```python
from build123d import *

# Parameters (mm, degrees)
SKETCH1_R           = 20
BOSS_EXTRUDE1_DEPTH = 35
CUT_EXTRUDE1_DEPTH  = 15
SKETCH3_R           = 4.1
CUT_EXTRUDE2_DEPTH  = 21
SKETCH4_R           = 2
CUT_EXTRUDE3_DEPTH  = 36
SKETCH5_R           = 17
CUT_EXTRUDE4_DEPTH  = 5


with BuildPart() as part:
    # Sketch1 → Boss-Extrude1 (new body)
    with BuildSketch(Plane(origin=(0, 0, 0), x_dir=(1, 0, 0), z_dir=(0, 1, 0))):
        Circle(SKETCH1_R)
    extrude(amount=BOSS_EXTRUDE1_DEPTH)

    # Sketch2 → Cut-Extrude1 (cut)
    with BuildSketch(Plane(origin=(0, 35, 0), x_dir=(1, 0, 0), z_dir=(0, 1, 0))):
        Polygon((-8, 7.5), (-14.495190528, 3.75), (-14.495190528, -3.75), (-8, -7.5), (-1.504809472, -3.75), (-1.504809472, 3.75), align=None)
        Polygon((8, 7.5), (1.504809472, 3.75), (1.504809472, -3.75), (8, -7.5), (14.495190528, -3.75), (14.495190528, 3.75), align=None)
    extrude(amount=-CUT_EXTRUDE1_DEPTH, mode=Mode.SUBTRACT)

    # Sketch3 → Cut-Extrude2 (cut, through all)
    with BuildSketch(Plane(origin=(0, 20, 0), x_dir=(1, 0, 0), z_dir=(0, 1, 0))):
        with Locations((-8, 0)):
            Circle(SKETCH3_R)
        with Locations((8, 0)):
            Circle(SKETCH3_R)
    extrude(amount=-CUT_EXTRUDE2_DEPTH, mode=Mode.SUBTRACT)

    # Sketch4 → Cut-Extrude3 (cut, through all)
    with BuildSketch(Plane(origin=(0, 35, 0), x_dir=(1, 0, 0), z_dir=(0, 1, 0))):
        with Locations((-10.5, 10.5)):
            Circle(SKETCH4_R)
        with Locations((10.5, 10.5)):
            Circle(SKETCH4_R)
        with Locations((10.5, -10.5)):
            Circle(SKETCH4_R)
        with Locations((-10.5, -10.5)):
            Circle(SKETCH4_R)
    extrude(amount=-CUT_EXTRUDE3_DEPTH, mode=Mode.SUBTRACT)

    # Sketch5 → Cut-Extrude4 (cut)
    with BuildSketch(Plane(origin=(0, 35, 0), x_dir=(1, 0, 0), z_dir=(0, 1, 0))):
        Circle(SKETCH5_R)
    extrude(amount=-CUT_EXTRUDE4_DEPTH, mode=Mode.SUBTRACT)


solid = part.part
```
CAD build for the part. Positions are in the model's coordinates, mm. A direction names the side the tool comes from. Coordinates: 2 decimals unless noted, no trailing zeros. Loops run counter-clockwise (first coordinate to the right, second up) from the corner with the lowest first, then second, coordinate; pieces in that order, holes last. Notation, with made-up numbers: (31, 40.25) - (78, 40.25) arc R23 ccw to (78, 62.25) - close; hole circle Ø7 at (40, -30.5). An arc over 180 degrees is marked (long way). Return JSON: item names as keys, results as strings.
1. Drop flat-ended pins along their axis: pin 1 (10.5 mm diameter, centred on x = -9, z = 3, fed in from +Y); pin 2 (1 mm diameter, centred on x = 9.5, y = 5.5, fed in from +Z); pin 3 (4 mm diameter, centred on x = 9.5, z = 3.5, fed in from +Y). Give the stop position or say it passes through.
Result:
{"pin 1": "stops at y = 30", "pin 2": "stops at z = 17.86", "pin 3": "stops at y = 20"}
2. Band-saw the part on C-C (x = 6). Give the cut face in (y, z), and give its area (3 significant figures).
Result:
{"outline": "(0, -19.08) - (35, -19.08) - (35, -15.91) - (30, -15.91) - (30, -6.35) - (20, -6.35) - (20, -3.58) - (0, -3.58) - close; (0, 3.58) - (20, 3.58) - (20, 6.35) - (30, 6.35) - (30, 15.91) - (35, 15.91) - (35, 19.08) - (0, 19.08) - close", "area": "906 mm2"}
3. Probe L1, parallel to Z at x = -10, y = 24.5; L2, parallel to X at y = 11.25, z = -10.5; L3, parallel to X at y = 33, z = 0. List the from-to ranges inside material, lowest first. Write a range as from..to.
Result:
{"L1": "z = -17.32..-12.44, -8.56..-6.35, 6.35..8.56, 12.44..17.32", "L2": "x = -17.02..-12.5, -8.5..8.5, 12.5..17.02", "L3": "x = -20..-17, 17..20"}
4. Band-saw the part on A-A (z = 0). Give the cut face in (x, y), and give its area (3 significant figures).
Result:
{"outline": "(-20, 0) - (-12.1, 0) - (-12.1, 20) - (-14.5, 20) - (-14.5, 30) - (-17, 30) - (-17, 35) - (-20, 35) - close; (-3.9, 0) - (3.9, 0) - (3.9, 20) - (1.5, 20) - (1.5, 30) - (-1.5, 30) - (-1.5, 20) - (-3.9, 20) - close; (12.1, 0) - (20, 0) - (20, 35) - (17, 35) - (17, 30) - (14.5, 30) - (14.5, 20) - (12.1, 20) - close", "area": "642 mm2"}
5. Band-saw the part on D-D (x = 0). Give the cut face in (y, z), and give its area (3 significant figures).
Result:
{"outline": "(0, -20) - (35, -20) - (35, -17) - (30, -17) - (30, 17) - (35, 17) - (35, 20) - (0, 20) - close", "area": "1,230 mm2"}
6. Band-saw the part on B-B (y = 8.5). Give the cut face in (x, z).
Result:
{"outline": "circle Ø40 at (0, 0); hole circle Ø4 at (-10.5, -10.5); hole circle Ø4 at (-10.5, 10.5); hole circle Ø8.2 at (-8, 0); hole circle Ø8.2 at (8, 0); hole circle Ø4 at (10.5, -10.5); hole circle Ø4 at (10.5, 10.5)"}
7. Mould opens along X. For faces 1 (the flat face through (11.29, 25.07, -5.6)), 2 (the flat face through (4.798, 25.07, -5.651)), 3 (the flat face through (0, 0, 0)) say: released by +X, released by -X, zero draft, split by the parting line, or undercut.
Result:
{"face 1": "undercut", "face 2": "undercut", "face 3": "zero draft"}
8. 3-axis set-ups, long thin cutter, end or side, ignore diameter. For faces 4 (the cylindrical face through (-11.974, 15.21, 9.148)), 5 (the flat face through (-14.495, 25, 0)): which of +Z, -Z, +X, -X, +Y, -Y reach the whole face in a straight line?
Result:
{"face 4": "+Y, -Y", "face 5": "+Y"}
